from build123d import *

# Parameters (mm, degrees)
SKETCH1_R                = 57.5
SKETCH1_R_2              = 45
BOSS_EXTRUDE1_DEPTH      = 13
BOSS_EXTRUDE2_START      = 1
SKETCH2_R                = 57.5
SKETCH2_R_2              = 45
BOSS_EXTRUDE2_DEPTH      = 1
BOSS_EXTRUDE3_START      = 2
SKETCH3_R                = 57.5
SKETCH3_R_2              = 42.5
BOSS_EXTRUDE3_DEPTH      = 2
SKETCH5_R                = 3
CUT_EXTRUDE2_DEPTH       = 13
FILLET4_R                = 0.5
SKETCH10_R               = 57.5
SKETCH10_R_2             = 45
BOSS_EXTRUDE4_DEPTH      = 1
SKETCH11_R               = 57.5
SKETCH11_R_2             = 42.5
BOSS_EXTRUDE5_DEPTH      = 2
SKETCH7_R                = 1.75
CUT_EXTRUDE3_DEPTH       = 23
CIRPATTERN3_COUNT        = 31
FILLET4_OF_CIRPATTERN3_R = 0.5
SKETCH4_R                = 1.75
CUT_EXTRUDE1_DEPTH       = 51
SKETCH14_R               = 84.700123292
CUT_EXTRUDE4_DEPTH       = 54


with BuildPart() as part:
    # Sketch1 → Boss-Extrude1 (new body)
    with BuildSketch(Plane(origin=(0, 0, 0), x_dir=(1, 0, 0), z_dir=(0, 1, 0))):
        with Locations(Location((0, 0, 0), (0, 0, 90))):
            Circle(SKETCH1_R)
        with Locations(Location((0, 0, 0), (0, 0, 90))):
            Circle(SKETCH1_R_2, mode=Mode.SUBTRACT)
    extrude(amount=BOSS_EXTRUDE1_DEPTH)

    # Sketch2 → Boss-Extrude2 (add)
    with BuildSketch(Plane.XZ.offset(BOSS_EXTRUDE2_START)):
        with Locations(Location((0, 0, 0), (0, 0, 270))):
            Circle(SKETCH2_R)
        with Locations(Location((0, 0, 0), (0, 0, 270))):
            Circle(SKETCH2_R_2, mode=Mode.SUBTRACT)
    extrude(amount=-BOSS_EXTRUDE2_DEPTH)

    # Sketch3 → Boss-Extrude3 (add)
    with BuildSketch(Plane.XZ.offset(1).offset(BOSS_EXTRUDE3_START)):
        with Locations(Location((0, 0, 0), (0, 0, 270))):
            Circle(SKETCH3_R)
        with Locations(Location((0, 0, 0), (0, 0, 270))):
            Circle(SKETCH3_R_2, mode=Mode.SUBTRACT)
    extrude(amount=-BOSS_EXTRUDE3_DEPTH)

    # Sketch5 → Cut-Extrude2 (cut)
    with BuildSketch(Plane(origin=(0, 13, 0), x_dir=(1, 0, 0), z_dir=(0, 1, 0))):
        with Locations((0, 45)):
            Circle(SKETCH5_R)
    cut_extrude2 = extrude(amount=-CUT_EXTRUDE2_DEPTH, mode=Mode.SUBTRACT)

    # Fillet4
    fillet4_edges = [part.edges().sort_by_distance(p)[0] for p in [
        (2.99833287, 6.5, -44.9),
        (-2.99833287, 6.5, -44.9),
    ]]
    fillet(fillet4_edges, radius=FILLET4_R)

    # Sketch10 → Boss-Extrude4 (add)
    with BuildSketch(Plane(origin=(0, 13, 0), x_dir=(1, 0, 0), z_dir=(0, 1, 0))):
        with Locations(Location((0, 0, 0), (0, 0, 90))):
            Circle(SKETCH10_R)
        with Locations(Location((0, 0, 0), (0, 0, 90))):
            Circle(SKETCH10_R_2, mode=Mode.SUBTRACT)
    extrude(amount=BOSS_EXTRUDE4_DEPTH)

    # Sketch11 → Boss-Extrude5 (add)
    with BuildSketch(Plane(origin=(0, 14, 0), x_dir=(1, 0, 0), z_dir=(0, 1, 0))):
        with Locations(Location((0, 0, 0), (0, 0, 90))):
            Circle(SKETCH11_R)
        with Locations(Location((0, 0, 0), (0, 0, 90))):
            Circle(SKETCH11_R_2, mode=Mode.SUBTRACT)
    extrude(amount=BOSS_EXTRUDE5_DEPTH)

    # Sketch7 → Cut-Extrude3 (cut)
    with BuildSketch(Plane(origin=(0, 16, 0), x_dir=(1, 0, 0), z_dir=(0, 1, 0))):
        with Locations(Location((0, 45, 0), (0, 0, 270))):
            Circle(SKETCH7_R)
    cut_extrude3 = extrude(amount=-CUT_EXTRUDE3_DEPTH, mode=Mode.SUBTRACT)

    # CirPattern3: Cut-Extrude2, Cut-Extrude3 ×31 about axis
    cirpattern3_axis = Axis((0, 0, 0), (0, 1, 0))
    add([cut_extrude2.rotate(cirpattern3_axis, i * 360 / CIRPATTERN3_COUNT) for i in range(1, CIRPATTERN3_COUNT)], mode=Mode.SUBTRACT)
    add([cut_extrude3.rotate(cirpattern3_axis, i * 360 / CIRPATTERN3_COUNT) for i in range(1, CIRPATTERN3_COUNT)], mode=Mode.SUBTRACT)

    # Fillet4 of CirPattern3
    fillet4_of_cirpattern3_edges = [part.edges().sort_by_distance(p)[0] for p in [
        (-6.101346732, 6.5, -44.584454332),
        (-11.975260372, 6.5, -43.377334393),
        (-14.951236482, 6.5, -42.443615865),
        (-20.461919307, 6.5, -40.078795619),
        (-23.189020853, 6.5, -38.565130777),
        (-28.110864862, 6.5, -35.139426243),
        (-30.477443987, 6.5, -33.107784704),
        (-34.608948306, 6.5, -28.761444629),
        (-36.518116982, 6.5, -26.295002036),
        (-39.690137341, 6.5, -21.205966091),
        (-41.063733978, 6.5, -18.405698895),
        (-43.146407489, 6.5, -12.782312811),
        (-43.92819688, 6.5, -9.762864278),
        (-44.836258645, 6.5, -3.835350142),
        (-44.99423424, 6.5, -0.720336851),
        (-44.690508104, 6.5, 5.268632212),
        (-44.218202364, 6.5, 8.351681252),
        (-42.715122911, 6.5, 14.156916145),
        (-41.631872087, 6.5, 17.081780543),
        (-38.990975566, 6.5, 22.465614267),
        (-37.341128076, 6.5, 25.112549731),
        (-33.670533101, 6.5, 29.854567501),
        (-31.521633894, 6.5, 32.115208183),
        (-26.971615054, 6.5, 36.021271235),
        (-24.411640317, 6.5, 37.803066239),
        (-19.168475919, 6.5, 40.713259891),
        (-16.302231317, 6.5, 41.943262321),
        (-10.580577126, 6.5, 43.738442904),
        (-7.525407051, 6.5, 44.366296315),
        (-1.559508263, 6.5, 44.972968926),
        (1.559508263, 6.5, 44.972968926),
        (7.525407051, 6.5, 44.366296315),
        (10.580577126, 6.5, 43.738442904),
        (16.302231317, 6.5, 41.943262321),
        (19.168475919, 6.5, 40.713259891),
        (24.411640317, 6.5, 37.803066239),
        (26.971615054, 6.5, 36.021271235),
        (31.521633894, 6.5, 32.115208183),
        (33.670533101, 6.5, 29.854567501),
        (37.341128076, 6.5, 25.112549731),
        (38.990975566, 6.5, 22.465614267),
        (41.631872087, 6.5, 17.081780543),
        (42.715122911, 6.5, 14.156916145),
        (44.218202364, 6.5, 8.351681252),
        (44.690508104, 6.5, 5.268632212),
        (44.99423424, 6.5, -0.720336851),
        (44.836258645, 6.5, -3.835350142),
        (43.92819688, 6.5, -9.762864278),
        (43.146407489, 6.5, -12.782312811),
        (41.063733978, 6.5, -18.405698895),
        (39.690137341, 6.5, -21.205966091),
        (36.518116982, 6.5, -26.295002036),
        (34.608948306, 6.5, -28.761444629),
        (30.477443987, 6.5, -33.107784704),
        (28.110864862, 6.5, -35.139426243),
        (23.189020853, 6.5, -38.565130777),
        (20.461919307, 6.5, -40.078795619),
        (14.951236482, 6.5, -42.443615865),
        (11.975260372, 6.5, -43.377334393),
        (6.101346732, 6.5, -44.584454332),
    ]]
    fillet(fillet4_of_cirpattern3_edges, radius=FILLET4_OF_CIRPATTERN3_R)

    # Sketch4 → Cut-Extrude1 (cut)
    with BuildSketch(Plane(origin=(0, 16, 0), x_dir=(1, 0, 0), z_dir=(0, 1, 0))):
        with Locations(Location((0, 54, 0), (0, 0, 270))):
            Circle(SKETCH4_R)
        with Locations(Location((20.664905348, 49.889494756, 0), (0, 0, 270))):
            Circle(SKETCH4_R)
        with Locations(Location((38.183766184, 38.183766184, 0), (0, 0, 270))):
            Circle(SKETCH4_R)
        with Locations(Location((49.889494756, 20.664905348, 0), (0, 0, 270))):
            Circle(SKETCH4_R)
        with Locations(Location((54, 0, 0), (0, 0, 270))):
            Circle(SKETCH4_R)
        with Locations(Location((49.889494756, -20.664905348, 0), (0, 0, 270))):
            Circle(SKETCH4_R)
        with Locations(Location((38.183766184, -38.183766184, 0), (0, 0, 270))):
            Circle(SKETCH4_R)
        with Locations(Location((20.664905348, -49.889494756, 0), (0, 0, 270))):
            Circle(SKETCH4_R)
        with Locations(Location((0, -54, 0), (0, 0, 270))):
            Circle(SKETCH4_R)
        with Locations(Location((-20.664905348, -49.889494756, 0), (0, 0, 270))):
            Circle(SKETCH4_R)
        with Locations(Location((-38.183766184, -38.183766184, 0), (0, 0, 270))):
            Circle(SKETCH4_R)
        with Locations(Location((-49.889494756, -20.664905348, 0), (0, 0, 270))):
            Circle(SKETCH4_R)
        with Locations(Location((-54, 0, 0), (0, 0, 270))):
            Circle(SKETCH4_R)
        with Locations(Location((-49.889494756, 20.664905348, 0), (0, 0, 270))):
            Circle(SKETCH4_R)
        with Locations(Location((-38.183766184, 38.183766184, 0), (0, 0, 270))):
            Circle(SKETCH4_R)
        with Locations(Location((-20.664905348, 49.889494756, 0), (0, 0, 270))):
            Circle(SKETCH4_R)
    extrude(amount=-CUT_EXTRUDE1_DEPTH, mode=Mode.SUBTRACT)

    # Sketch14 → Cut-Extrude4 (cut)
    with BuildSketch(Plane(origin=(0, 0, 0), x_dir=(1, 0, 0), z_dir=(0, 1, 0))):
        Circle(SKETCH14_R)
    extrude(amount=CUT_EXTRUDE4_DEPTH, mode=Mode.SUBTRACT)


solid = part.part
For this review, take the finished solid that the model builds, in its own axes (mm). A direction names the side the tool comes from. Coordinates: 2 decimals unless noted, no trailing zeros. Loops run counter-clockwise (first coordinate to the right, second up) from the corner with the lowest first, then second, coordinate; pieces in that order, holes last. Notation, with made-up numbers: (60.5, 45) -> (69.5, 45) arc R26 cw to (69.5, 75) -> close; hole circle Ø3 at (13, 32.5). An arc over 180 degrees is marked (long way). Write each question's results on one line, items separated by ' | '.
Q1. Add section C-C, the plane x = 54. State the section outline as (y, z) points, then the cut area to 3 significant figures.
Taken from the geometry:
outline: (-3, -19.75) -> (0, -19.75) -> (0, -1.75) -> (-3, -1.75) -> close; (-3, 1.75) -> (0, 1.75) -> (0, 19.75) -> (-3, 19.75) -> close | area: 108 mm²
Q2. Add section A-A, the plane x = 0. State the section outline as (y, z) points, then the cut area to 4 significant figures.
Taken from the geometry:
outline: (-3, -57.5) -> (0, -57.5) -> (0, -55.75) -> (-3, -55.75) -> close; (-3, -52.25) -> (0, -52.25) -> (0, -46.75) -> (-3, -46.75) -> close; (-3, -43.25) -> (-1, -43.25) -> (-1, -42.5) -> (-3, -42.5) -> close; (-3, 42.5) -> (-1, 42.5) -> (-1, 45) -> (0, 45) -> (0, 52.25) -> (-3, 52.25) -> close; (-3, 55.75) -> (0, 55.75) -> (0, 57.5) -> (-3, 57.5) -> close | area: 55.25 mm²
Q3. Machinability: for faces 1 (the cylindrical face through (-39.632, -1.812, -24.793)), 2 (the flat face through (30.2, -1, 30.2)), which of the approach directions +Z, -Z, +X, -X, +Y, -Y give a long, thin tool a straight path to every point of the face, cutting with its end or side? Answer none if there is none.
Taken from the geometry:
face 1: +Y, -Y | face 2: +Y
Q4. To check wall thickness, follow line 1 along Z through (x, y) = (-7.5, -1.1); line 2 along Z through (x, y) = (14.5, -1.95); line 3 along Z through (x, y) = (21, -1.9). State the ranges of each line that lie inside material, in increasing order. Write a range as [from, to].
Taken from the geometry:
line 1: [-57.01, -44.87], [-43.28, -41.83], [41.83, 57.01] | line 2: [-55.64, -39.95], [39.95, 41.52], [44.35, 55.64] | line 3: [-53.53, -51.61], [-48.17, -36.95], [36.95, 37.81], [40.88, 48.17], [51.61, 53.53]
Q5. Add section B-B, the plane z = 54. State the section outline as (x, y) points.
Taken from the geometry:
outline: (-19.75, -3) -> (-1.75, -3) -> (-1.75, 0) -> (-19.75, 0) -> close; (1.75, -3) -> (19.75, -3) -> (19.75, 0) -> (1.75, 0) -> close
Q6. Add section D-D, the plane y = -2.35. Count the separate pieces of the cut face and the enclosed holes in it, then the cut area to 3 significant figures.
Taken from the geometry:
separate pieces: 1 | enclosed holes: 48 | area: 4,260 mm²
Q7. For pin 1 Ø1 at (y, z) = (-2, 26) entering from -X; pin 2 Ø1.5 at (x, y) = (-24, -1.5) entering from +Z, all flat-tipped, find the tip position at first contact; note any pin that passes through.
Taken from the geometry:
pin 1: x = -51.54 | pin 2: z = 52.59
